from build123d import *
from build123d.topology import SkipClean

# Parameters (mm, degrees)
EXTRUDE_1_DEPTH     = 3
SKETCH_2_R          = 2
SKETCH_2_R_2        = 1.9999999999999967
CUT_EXTRUDE_1_DEPTH = 105.01455903133225
EXTRUDE_START       = 3
SKETCH_3_R          = 1.9999999999999962
SKETCH_3_R_2        = 2
EXTRUDE_9_DEPTH     = 3
FILLET_1_R          = 10
FILLET_2_R          = 10


with BuildPart() as part:
    # 草图1 → 凸台-拉伸1 (new body)
    with BuildSketch(Plane.XY):
        with BuildLine():
            Line((21.79390335077292, -7.475214596472519), (7.229933319640558, 1.9945085092702048))
            ThreePointArc((7.229933319640558, 1.9945085092702048), (-6.483154274799016, 3.7707705643747733), (1.8411668544431816, -7.270495486148093))
            Line((1.8411668544431845, -7.270495486148092), (14.486878939127898, -15.510906506800303))
            Line((14.486878939127898, -15.510906506800302), (82.06831155956868, -15.510906506800302))
            Line((82.06831155956867, -15.510906506800302), (96.3582789784704, -6.83317051644414))
            ThreePointArc((96.35827897847041, -6.833170516444138), (100.33032000817497, 6.162825901013469), (87.812990018917, 0.8723171575890092))
            Line((87.81299001891699, 0.8723171575890003), (74.06678283695699, -7.475214596472519))
            Line((74.06678283695699, -7.475214596472519), (21.79390335077292, -7.475214596472519))
        make_face()
    extrude(amount=EXTRUDE_1_DEPTH)

    # 草图2 → 切除-拉伸1 (cut, through all)
    with BuildSketch(Plane.XY.offset(3)):
        Circle(SKETCH_2_R)
        with Locations((95.30778311888552, 0.5928956325337316)):
            Circle(SKETCH_2_R_2)
    extrude(amount=-CUT_EXTRUDE_1_DEPTH, mode=Mode.SUBTRACT)

    # 草图3 → 凸台-拉伸9 (add)
    # profile 1 of 3: a face of its own
    with SkipClean():  # the faces are left unmerged after this step: merging them gives an invalid solid
        with BuildSketch(Plane(origin=(0, 0, 0), x_dir=(-1, 0, 0), z_dir=(0, 0, -1)).offset(EXTRUDE_START)):
            with BuildLine():
                ThreePointArc((-91.01590945402396, -5.557699496790565), (-89.75367146553334, -4.447128548171897), (-88.77053253167215, -3.0832918980444344))
                ThreePointArc((-88.77053253167215, -3.0832918980444344), (-88.05246164412989, -1.3071860230668506), (-87.80778311888552, 0.5928956325337297))
                ThreePointArc((-87.80778311888552, 0.5928956325337316), (-87.80908495687888, 0.7326306500420054), (-87.812990018917, 0.8723171575890011))
                ThreePointArc((-87.81299001891699, 0.8723171575890014), (-100.33032000817497, 6.162825901013491), (-96.35827897847041, -6.833170516444131))
                ThreePointArc((-96.35827897847042, -6.833170516444138), (-93.56613473312304, -6.702079412000068), (-91.01590945402396, -5.557699496790565))
            make_face()
            with Locations(Location((-95.30778311888552, 0.5928956325337316, 0), (0, 0, 180))):
                Circle(SKETCH_3_R, mode=Mode.SUBTRACT)
        # profile 2 of 3: a face of its own
        with BuildSketch(Plane(origin=(0, 0, 0), x_dir=(-1, 0, 0), z_dir=(0, 0, -1)).offset(EXTRUDE_START)):
            with BuildLine():
                Line((-75.05143042110615, -10.798154811245045), (-88.77053253167215, -3.0832918980444335))
                ThreePointArc((-88.77053253167215, -3.0832918980444344), (-89.75367146553334, -4.447128548171897), (-91.01590945402396, -5.557699496790565))
                Line((-91.01590945402396, -5.557699496790569), (-76.64805579661679, -13.637384335527532))
                Line((-76.64805579661679, -13.637384335527532), (-18.81509472588799, -13.637384335527532))
                Line((-18.81509472588799, -13.637384335527532), (-4.475261433860523, -6.018474482674216))
                ThreePointArc((-4.475261433860524, -6.018474482674214), (-5.688218997555007, -4.8881657741789315), (-6.623200748856248, -3.5189788064650287))
                Line((-6.623200748856245, -3.5189788064650287), (-20.323608343622624, -10.798154811245045))
                Line((-20.323608343622624, -10.798154811245045), (-75.05143042110615, -10.798154811245045))
            make_face()
        # profile 3 of 3: a face of its own
        with BuildSketch(Plane(origin=(0, 0, 0), x_dir=(-1, 0, 0), z_dir=(0, 0, -1)).offset(EXTRUDE_START)):
            with BuildLine():
                ThreePointArc((-7.229933319640558, 1.9945085092702044), (-7.454996074789714, -0.8203862047048063), (-6.623200748856248, -3.5189788064650287))
                ThreePointArc((-6.623200748856248, -3.5189788064650287), (-5.688218997555007, -4.8881657741789315), (-4.475261433860524, -6.018474482674214))
                ThreePointArc((-4.475261433860524, -6.018474482674214), (-3.2196592565993294, -6.773757765922417), (-1.8411668544431843, -7.270495486148093))
                ThreePointArc((-1.8411668544431843, -7.270495486148093), (4.606584884254069, -5.918561962517747), (7.5, -1.84e-15))
                ThreePointArc((7.5, 0), (1.00635483371816, 7.432176662906506), (-7.229933319640558, 1.9945085092702044))
            make_face()
            with Locations(Location((0, 0, 0), (0, 0, 180))):
                Circle(SKETCH_3_R_2, mode=Mode.SUBTRACT)
        extrude(amount=-EXTRUDE_9_DEPTH)

    # 圆角1
    # the kernel refuses this fillet: 10 mm, written as the material it adds along each edge
    with BuildSketch(Plane(origin=(88.77053253167215, -3.083291898044434, -3), x_dir=(-0.20664882712832097, 0.9784151788716738, 0), z_dir=(0, 0, 1))) as fillet_1_piece_1_section:
        with BuildLine():
            CenterArc((7.4864083793494025, 9.541100058820126), FILLET_1_R, 197.4249522895106, 55.15009542096897)
            Line((-2.0546916794712278, 6.546536707082027), (0, 0))
            ThreePointArc((0, 0), (2.245922513804829, 0.34417495588492364), (4.491845027609668, -5e-17))
        make_face()
    fillet_1_piece_1 = extrude(amount=20.153516540869376, mode=Mode.PRIVATE)
    fillet_1_piece_1 = split(fillet_1_piece_1, bisect_by=Plane(origin=(86.96414266235654, -3.033123271198268, 3), z_dir=(0, 0, -1)), keep=Keep.TOP, mode=Mode.PRIVATE)
    add(fillet_1_piece_1)
    with BuildSketch(Plane(origin=(91.01590945402396, -5.557699496790567, -3), x_dir=(0.9194568899378542, -0.39319082841008474, 0), z_dir=(0, 0, 1))) as fillet_1_piece_2:
        with BuildLine():
            CenterArc((5.092784059285759, -9.790309907458374), FILLET_1_R, 101.75407382431756, 40.75010367707175)
            Line((-2.8411931775201964, -3.7032740766253633), (0, 0))
            ThreePointArc((0, 0), (1.5278352177857282, -0.1572675694062238), (3.055670435571466, 9e-17))
        make_face()
    extrude(amount=3)
    with BuildSketch(Plane(origin=(4.475261433860524, -6.018474482674215, -3), x_dir=(-0.9077280584793651, -0.4195590206982592, 0), z_dir=(0, 0, 1))) as fillet_1_piece_3_section:
        with BuildLine():
            CenterArc((5.124050374991801, 9.787699282299565), FILLET_1_R, 217.21105425538934, 40.96167029208499)
            Line((-2.840082184875719, 3.740171475926284), (0, 0))
            ThreePointArc((0, 0), (1.53721511249754, 0.15922553827532712), (3.0744302249950772, 4e-17))
        make_face()
    fillet_1_piece_3 = extrude(amount=14.740674354083392, mode=Mode.PRIVATE)
    fillet_1_piece_3 = split(fillet_1_piece_3, bisect_by=Plane(origin=(4.991537565692553, -6.857429506035165, 3), z_dir=(0, 0, -1)), keep=Keep.TOP, mode=Mode.PRIVATE)
    add(fillet_1_piece_3)
    with BuildSketch(Plane(origin=(6.623200748856247, -3.5189788064650287, -3), x_dir=(0.883093433180833, -0.46919717419533746, 0), z_dir=(0, 0, 1))) as fillet_1_piece_4:
        with BuildLine():
            CenterArc((6.861406616347785, 10.000000000000002), FILLET_1_R, 214.84990457904146, 55.15009542095851)
            ThreePointArc((-1.3451114501356154, 4.285714285715009), (-0.3441749558850217, 2.245922513805171), (0, 0))
            Line((0, 0), (6.861406616347784, -2e-17))
        make_face()
    extrude(amount=3)

    # 圆角2
    fillet_2_edges = [part.edges().sort_by_distance(p)[0] for p in [
        (21.79390335077292, -7.475214596472519, 1.5),
        (74.06678283695699, -7.475214596472519, 1.5),
        (82.06831155956868, -15.510906506800302, 1.5),
        (14.486878939127898, -15.510906506800303, 1.5),
        (76.64805579661679, -13.637384335527532, -1.5),
        (18.81509472588799, -13.637384335527532, -1.5),
        (20.323608343622624, -10.798154811245045, -1.5),
        (75.05143042110615, -10.798154811245045, -1.5),
    ]]
    fillet(fillet_2_edges, radius=FILLET_2_R)


solid = part.part
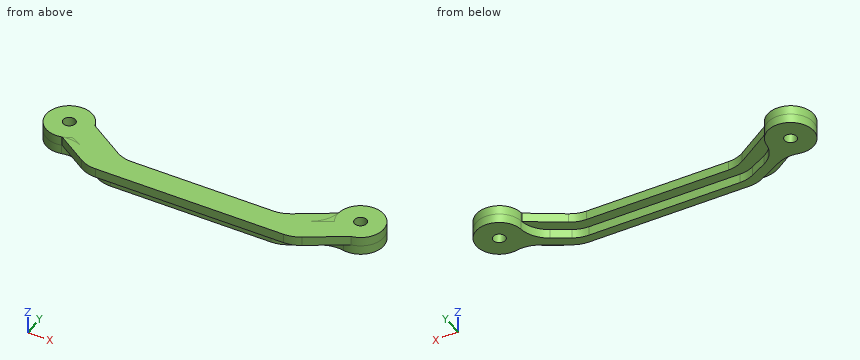
Verification items for the finished model (mm, model axes). Round coordinates to 2 decimals unless told otherwise and drop trailing zeros. Write each loop counter-clockwise with the first axis right and the second up, starting at its lowest first coordinate (ties: lowest second). Pieces come first, ordered by that corner, then holes.
(1) Section check C-C (z = 1.75). Enter the section's corners in (x, y).
Returned:
outline: (1.68, -7.31) arc R10 cw to (1.84, -7.27) - (12, -13.89) arc R10 ccw to (17.46, -15.51) - (79.27, -15.51) arc R10 ccw to (84.46, -14.06) - (96.36, -6.83) arc R7.5 ccw (long way) to (87.84, 1.31) arc R10 cw to (87.79, 0.86) - (76.46, -6.02) arc R10 cw to (71.27, -7.48) - (24.76, -7.48) arc R10 cw to (19.31, -5.86) - (7.23, 1.99) arc R7.5 ccw (long way) to start; hole circle Ø4 at (0, 0); hole circle Ø4 at (95.31, 0.59)
(2) Section check A-A (x = 0). Enter the section's corners in (y, z).
Returned:
outline: (-7.5, -3) - (-2, -3) - (-2, 3) - (-7.5, 3) - close; (2, -3) - (7.5, -3) - (7.5, 3) - (2, 3) - close
(3) Material ranges on line 1 (X direction, y = 1.75, z = -2.25); line 2 (X direction, y = 2.25, z = 1); line 3 (Y direction, x = 33.5, z = 0.75), recorded low to high.
Returned:
line 1: x = -7.29 to -0.97, 0.97 to 7.29, 87.9 to 93.68, 96.94 to 102.72
line 2: x = -7.15 to 7.15, 87.99 to 94.19, 96.43 to 102.62
line 3: y = -15.51 to -7.48
(4) Section check D-D (x = 14.5). Enter the section's corners in (y, z), plus the area to 3 significant figures.
Returned:
outline: (-15.06, 0) - (-11.34, 0) - (-11.34, -3) - (-7.7, -3) - (-7.7, 0) - (-2.73, 0) - (-2.73, 3) - (-15.06, 3) - close
area: 47.9 mm2
(5) Section check B-B (x = 38). Enter the section's corners in (y, z).
Returned:
outline: (-15.51, 0) - (-13.64, 0) - (-13.64, -3) - (-10.8, -3) - (-10.8, 0) - (-7.48, 0) - (-7.48, 3) - (-15.51, 3) - close
(6) Depth check by flat-ended pin: pin 1 Ø1.5 at (x, z) = (57, -1) entering from -Y; pin 2 Ø0.9 at (x, z) = (47, -2) entering from +Y; pin 3 Ø2.5 at (x, y) = (0, 0) entering from -Z; pin 4 Ø4 at (x, y) = (30, -7.5) entering from -Z. Enter the tip coordinate at first touch or a pass-through.
Returned:
pin 1: stops at y = -13.64
pin 2: stops at y = -10.8
pin 3: passes through
pin 4: stops at z = 0
